from build123d import *

# Parameters (mm, degrees)
SKETCH1_W             = 63.5
SKETCH1_H             = 59.69
BOSS_EXTRUDE1_DEPTH   = 3.0734
FILLET1_R             = 1.27
F_8_CLEARANCE_HOLE1_D = 4.4958
CUT_EXTRUDE1_DEPTH    = 4.0734
FILLET2_R             = 0.0635


with BuildPart() as part:
    # Sketch1 → Boss-Extrude1 (new body)
    with BuildSketch(Plane.XY):
        with Locations((31.75, 29.845)):
            Rectangle(SKETCH1_W, SKETCH1_H)
    extrude(amount=BOSS_EXTRUDE1_DEPTH)

    # Fillet1
    fillet1_edges = [part.edges().sort_by_distance(p)[0] for p in [
        (0, 59.69, 1.5367),
        (63.5, 59.69, 1.5367),
        (63.5, 0, 1.5367),
        (0, 0, 1.5367),
    ]]
    fillet(fillet1_edges, radius=FILLET1_R)

    # #8 Clearance Hole1 (through all)
    with Locations(Plane.XY.offset(3.0734)):
        with Locations((5.08, 54.61), (58.42, 54.61), (58.42, 5.08), (5.08, 5.08)):
            Hole(F_8_CLEARANCE_HOLE1_D / 2)

    # Sketch7 → Cut-Extrude1 (cut, through all)
    with BuildSketch(Plane.XY.offset(3.0734)):
        Polygon((31.242, 29.845), (31.242, 31.115), (30.734, 31.115), (31.75, 32.385), (32.766, 31.115), (32.258, 31.115), (32.258, 29.845), align=None)
    extrude(amount=-CUT_EXTRUDE1_DEPTH, mode=Mode.SUBTRACT)

    # Fillet2
    fillet2_edges = [part.edges().sort_by_distance(p)[0] for p in [
        (32.258, 29.845, 1.5367),
        (31.242, 29.845, 1.5367),
        (30.734, 31.115, 1.5367),
        (31.75, 32.385, 1.5367),
        (32.766, 31.115, 1.5367),
        (32.258, 31.115, 1.5367),
    ]]
    fillet(fillet2_edges, radius=FILLET2_R)


solid = part.part
Geometry: final body of the model. Coordinates: model frame, mm. Coordinates: 2 decimals unless noted, no trailing zeros. Write each loop counter-clockwise with the first axis right and the second up, starting at its lowest first coordinate (ties: lowest second). Pieces come first, ordered by that corner, then holes. Notation, with made-up numbers: (-13, 1) - (39, 1) arc R34 cw to (39, 31) - close; hole circle Ø8 at (44.5, 1.25). An arc over 180 degrees is marked (long way). Return JSON: item names as keys, results as strings.
Item 1: Line query: L1, parallel to Y at x = 5.08, z = 0.9; L2, parallel to X at y = 5, z = 2.8; L3, parallel to Y at x = 60, z = 1.65. Output: solid intervals per line, ascending.
Completed:
{"L1": "y = 0 to 2.83, 7.33 to 52.36, 56.86 to 59.69", "L2": "x = 0 to 2.83, 7.33 to 56.17, 60.67 to 63.5", "L3": "y = 0 to 3.48, 6.68 to 53.01, 56.21 to 59.69"}
Item 2: Pull-direction query (Y, two-part tool) for faces 1 (the face through (31, 59.69, 2)), 2 (the face through (56.344, 53.749, 1.515)), 3 (the face through (0, 29, 2)); classes: +Y half, -Y half, draft (parallel to the pull), parting line (faces both ways), or undercut.
Completed:
{"face 1": "+Y half", "face 2": "undercut", "face 3": "draft"}
Item 3: Section query A-A (z = 2.15). Count the separate pieces of the cut face and the enclosed holes in it, and give its area (3 significant figures).
Completed:
{"separate pieces": "1", "enclosed holes": "5", "area": "3,720 mm2"}
Item 4: Pin query (flat end, axial travel): pin 1 Ø5 at (x, y) = (5.08, 5.08) entering from -Z. Return the tip coordinate at first contact, or that it passes through.
Completed:
{"pin 1": "stops at z = 0"}
Item 5: Section query C-C (y = 5.08). Output: boundary loops of the cut face in (x, z).
Completed:
{"outline": "(0, 0) - (2.83, 0) - (2.83, 3.07) - (0, 3.07) - close; (7.33, 0) - (56.17, 0) - (56.17, 3.07) - (7.33, 3.07) - close; (60.67, 0) - (63.5, 0) - (63.5, 3.07) - (60.67, 3.07) - close"}
Item 6: Section query B-B (x = 58.42). Output: boundary loops of the cut face in (y, z), and give its area (3 significant figures).
Completed:
{"outline": "(0, 0) - (2.83, 0) - (2.83, 3.07) - (0, 3.07) - close; (7.33, 0) - (52.36, 0) - (52.36, 3.07) - (7.33, 3.07) - close; (56.86, 0) - (59.69, 0) - (59.69, 3.07) - (56.86, 3.07) - close", "area": "156 mm2"}
